CAD build for the part. Positions are in the model's coordinates, mm. A direction names the side the tool comes from. Round coordinates to 2 decimals unless told otherwise and drop trailing zeros. Write each loop counter-clockwise with the first axis right and the second up, starting at its lowest first coordinate (ties: lowest second). Pieces come first, ordered by that corner, then holes. Notation, with made-up numbers: M -13,55.5 L 41,55.5 A19 ccw 41,71.5 Z; hole C 51.25,32.5 d1. An arc over 180 degrees is marked long. Write each question's results on one line, items separated by ' | '. Start each with the question number.
```python
from build123d import *

# Parameters (mm, degrees)
BASE_DEPTH = 2.54


with BuildPart() as part:
    # Sketch1 → Base (new body)
    with BuildSketch(Plane(origin=(0, 0, 0), x_dir=(0, 0, -1), z_dir=(1, 0, 0))):
        with BuildLine():
            Line((-3, 0), (3, 0))
            Line((3, 0), (3, -2.54))
            Line((3, -2.54), (6.026607669, -2.54))
            ThreePointArc((6.026607669, -2.54), (0, -6.54), (-6.026607669, -2.54))
            Line((-6.026607669, -2.54), (-3, -2.54))
            Line((-3, -2.54), (-3, 0))
        make_face()
    extrude(amount=BASE_DEPTH)


solid = part.part
```
1) Drop flat-ended pins along their axis: pin 1 Ø1 at (x, y) = (2, -4.5) entering from +Z; pin 2 Ø1.3 at (x, z) = (1.5, -4) entering from +Y; pin 3 Ø1 at (x, y) = (2, -1) entering from -Z. Give the stop position or say it passes through.
2) Saw through at B-B, the plane y = -2. Write the cut outline in (x, z), plus the area to 3 significant figures.
3) Saw through at C-C, the plane z = -4.25. Write the cut outline in (x, y), plus the area to 3 significant figures.
4) Wall check: line 1 along Z through (x, y) = (1.4, -1.75); line 2 along Y through (x, z) = (2.1, 4); line 3 along Z through (x, y) = (1.35, -5.5). Give the ranges that are in metal, low to high. Write a range as from..to.
5) Saw through at A-A, the plane x = 2.15. Write the cut outline in (y, z).
6) 3-axis set-ups, long thin cutter, end or side, ignore diameter. For faces 1 (the face through (1, -1, -3)), 2 (the face through (1, -1, 3)), 3 (the face through (1.25, -6.54, -0.11)): which of +Z, -Z, +X, -X, +Y, -Y reach the whole face in a straight line?
Filled sheet:
1) pin 1: stops at z = 5.17 | pin 2: stops at y = -2.54 | pin 3: stops at z = -3
2) outline: M 0,-3 L 2.54,-3 L 2.54,3 L 0,3 Z | area: 15.2 mm^2
3) outline: M 0,-4.97 L 2.54,-4.97 L 2.54,-2.54 L 0,-2.54 Z | area: 6.17 mm^2
4) line 1: z = -3..3 | line 2: y = -5.17..-2.54 | line 3: z = -3.54..3.54
5) outline: M -2.54,-6.03 L -2.54,-3 L 0,-3 L 0,3 L -2.54,3 L -2.54,6.03 A6.54 ccw Z
6) face 1: -Z, +X, -X, +Y | face 2: +Z, +X, -X, +Y | face 3: +X, -X, -Y
